The listing builds one solid part. Answer for the finished solid, in the listing's coordinates (mm). A direction names the side the tool comes from. Coordinates: 2 decimals unless noted, no trailing zeros. Loops run counter-clockwise (first coordinate to the right, second up) from the corner with the lowest first, then second, coordinate; pieces in that order, holes last. Notation, with made-up numbers: (49, -1) - (72, -1) arc R30 cw to (72, 34) - close; hole circle Ø1 at (26, 11.25). An arc over 180 degrees is marked (long way). Return JSON: item names as keys, results as strings. Group by question number.
1. Section D-D (y = -57.15) is taken. Write down the section's boundary in (x, z).
2. Find the intervals of material crossed by line 1 along Y through (x, z) = (-8.75, 0) (3 decimals); line 2 along Y through (x, z) = (-14, 0); line 3 along Z through (x, y) = (18.2, 0), in increasing order.
3. Section B-B (z = 0) is taken. State how many separate pieces and enclosed holes the cut face has, and give its area (3 significant figures).
4. Each of these flat-tipped pins is pushed along its axis until it touches: P1, Ø20, axis at y = 0, z = 0, coming from the -X side; P2, Ø4, axis at x = 2.5, z = -11, coming from the -Y side; P3, Ø18, axis at y = 0, z = 0, coming from the +X side. Where does it stop, or does it pass through?
5. The mould has two halves that part along Y. Classify faces 5 (the face through (-13, -68.542, 0)), 6 (the face through (-19.05, 72, 0)), 7 (the face through (-17.641, -5.736, 11.028)): pulls with the +Y half, pulls with the -Y half, needs draft (parallel to the pull), parting line crosses it, or undercut.
6. Which of the six approach directions +Z, -Z, +X, -X, +Y, -Y give full straight-line access (tool end or side, diameter ignored) to faces 1 (the face through (-13.25, -6.04, -9.48)), 2 (the face through (-6.35, -50, 0)), 3 (the face through (0, 105, -19.05)), 4 (the face through (10.636, -0.2, 7.3))?
```python
from build123d import *

# Parameters (mm, degrees)
SKETCH5_W               = 38.1
SKETCH5_H               = 298.45
BOSS_EXTRUDE2_DEPTH     = 19.05
F_3_8_CLEARANCE_HOLE2_D = 10.0838
F_3_8_CLEARANCE_HOLE4_D = 13.97
BODY_MOVE_COPY4_ANGLE   = 90
CUT_EXTRUDE1_DEPTH      = 218.574389578
CUT_EXTRUDE1_DEPTH_BACK = 218.574389578
CUT_EXTRUDE5_DEPTH      = 218.574389578
CUT_EXTRUDE5_DEPTH_BACK = 218.574389578


with BuildPart() as part:
    # Sketch5 → Boss-Extrude2 (new, symmetric)
    with BuildSketch(Plane.XY):
        with Locations((0, 66.675)):
            Rectangle(SKETCH5_W, SKETCH5_H)
    extrude(amount=BOSS_EXTRUDE2_DEPTH, both=True)

    # 3/8 Clearance Hole2 (through all)
    with Locations(Plane(origin=(19.05, 0, 0), x_dir=(0, 0, -1), z_dir=(1, 0, 0))):
        with Locations((0, -57.15)):
            Hole(F_3_8_CLEARANCE_HOLE2_D / 2)

    # 3/8 Clearance Hole4 (through all)
    with Locations(Plane(origin=(19.05, 0, 0), x_dir=(0, 0, -1), z_dir=(1, 0, 0))):
        with Locations((0, 0)):
            Hole(F_3_8_CLEARANCE_HOLE4_D / 2)


with BuildPart() as body_2:
    # uxcell-FR6ZZ: read off the stored shape, not the designer's step
    # uxcell-FR6ZZ outline → uxcell-FR6ZZ (revolve)
    with BuildSketch(Plane(origin=(46.870492888, 0, -67.456601715), x_dir=(1, 0, 0), z_dir=(0, 0, 1))):
        Polygon((12.430125, 146.229545606), (4.7625, 146.229545606), (4.7625, 137.815795606), (11.2395, 137.815795606), (11.2395, 142.975170606), (11.636375, 143.372045606), (12.430125, 143.372045606), align=None)
    revolve(axis=Axis((46.870492888, 0, -67.456601715), (0, 1, 0)))


with BuildPart() as body_2_1:
    # Body-Move/Copy4: read off the stored shape, not the designer's step
    # Body-Move/Copy4: moved
    add(body_2.part.moved(Location((-46.8704929, -127.1795456, 67.4566017))).rotate(Axis((0, 0, 0), (0, 0, -1)), BODY_MOVE_COPY4_ANGLE))


with BuildPart() as body_3:
    # Mirror1: mirrored copy
    add(body_2_1.part.mirror(Plane(origin=(0, 0, 0), x_dir=(0, 0, 1), z_dir=(1, 0, 0))))


with BuildPart() as part_1:
    add(part.part)

    # Combine2: cut body 3, body 2
    add(body_3.part, mode=Mode.SUBTRACT)
    add(body_2_1.part, mode=Mode.SUBTRACT)

    # Sketch11 → Cut-Extrude1 (cut, two sides: drawn at the far end of the back side and taken through both)
    with BuildSketch(Plane.XY.offset(-CUT_EXTRUDE1_DEPTH_BACK)):
        Polygon((-6.35, -691.607801887), (-6.35, -82.55), (-6.35, -31.75), (19.05, -25.4), (609.922858655, 122.318214664), (1581.067185153, -612.994182394), (964.794326498, -1426.920198945), align=None)
    extrude(amount=CUT_EXTRUDE1_DEPTH + CUT_EXTRUDE1_DEPTH_BACK, mode=Mode.SUBTRACT)

    # Sketch18 → Cut-Extrude5 (cut, two sides: drawn at the far end of the back side and taken through both)
    with BuildSketch(Plane(origin=(0, 0, 0), x_dir=(0, 0, -1), z_dir=(1, 0, 0)).offset(-CUT_EXTRUDE5_DEPTH_BACK)):
        Polygon((-67.601886726, 453.814659538), (-19.05, -8.125685716), (-12.7, -68.5419), (12.7, -68.5419), (19.05, -8.125685716), (67.601886726, 453.814659538), (67.601886726, -475.155024096), (-67.601886726, -475.155024096), align=None)
    extrude(amount=CUT_EXTRUDE5_DEPTH + CUT_EXTRUDE5_DEPTH_BACK, mode=Mode.SUBTRACT)


solid = part_1.part
```
The answers:
{
 "1": {"outline": "(-19.05, -13.9) - (-6.35, -13.9) - (-6.35, -5.04) - (-19.05, -5.04) - close; (-19.05, 5.04) - (-6.35, 5.04) - (-6.35, 13.9) - (-19.05, 13.9) - close"},
 "2": {"line 1": "y = -68.542 to -62.192, -52.108 to -6.985, 6.985 to 215.9", "line 2": "y = -68.54 to -62.19, -52.11 to -11.24, 11.24 to 215.9", "line 3": "z = -19.05 to -12.43, 12.43 to 19.05"},
 "3": {"separate pieces": "3", "enclosed holes": "0", "area": "9,000 mm2"},
 "4": {"P1": "stops at x = -10.64", "P2": "stops at y = -30.04", "P3": "stops at x = 10.64"},
 "5": {"face 5": "pulls with the -Y half", "face 6": "needs draft", "face 7": "undercut"},
 "6": {"face 1": "-X", "face 2": "+Z, -Z, +X, -Y", "face 3": "-Z, +X, -X, +Y, -Y", "face 4": "+X"}
}
